```python
from build123d import *

# Parameters (mm, degrees)
SKETCH1_W           = 40
SKETCH1_H           = 25
BOSS_EXTRUDE1_DEPTH = 2
SKETCH2_W           = 25
SKETCH2_H           = 2
BOSS_EXTRUDE2_DEPTH = 2
SKETCH3_W           = 13
SKETCH3_H           = 17
CUT_EXTRUDE1_DEPTH  = 3
SKETCH4_R           = 0.6
BOSS_EXTRUDE3_DEPTH = 5
SKETCH5_W           = 16
SKETCH5_H           = 2
BOSS_EXTRUDE4_DEPTH = 4
SKETCH6_W           = 12
SKETCH6_H           = 2
CUT_EXTRUDE2_DEPTH  = 4
FILLET1_START       = -1
FILLET1_DEPTH       = 4
FILLET1_2_DEPTH     = 2
MIRROR4_DEPTH       = 2
FILLET2_R           = 2
FILLET3_R           = 2


with BuildPart() as part:
    # Sketch1 → Boss-Extrude1 (new body)
    with BuildSketch(Plane(origin=(0, 0, 0), x_dir=(1, 0, 0), z_dir=(0, 1, 0))):
        Rectangle(SKETCH1_W, SKETCH1_H)
    extrude(amount=BOSS_EXTRUDE1_DEPTH)

    # Sketch2 → Boss-Extrude2 (add)
    with BuildSketch(Plane(origin=(0, 2, 0), x_dir=(1, 0, 0), z_dir=(0, 1, 0))):
        with Locations((-7.5, 11.5)):
            Rectangle(SKETCH2_W, SKETCH2_H)
    boss_extrude2 = extrude(amount=BOSS_EXTRUDE2_DEPTH)

    # Mirror1: Boss-Extrude2 across plane
    add(boss_extrude2.mirror(Plane.XY))

    # Sketch3 → Cut-Extrude1 (cut)
    with BuildSketch(Plane(origin=(0, 2, 0), x_dir=(1, 0, 0), z_dir=(0, 1, 0))):
        with Locations((13.5, 0)):
            Rectangle(SKETCH3_W, SKETCH3_H)
    extrude(amount=-CUT_EXTRUDE1_DEPTH, mode=Mode.SUBTRACT)

    # Sketch4 → Boss-Extrude3 (add)
    with BuildSketch(Plane(origin=(0, 2, 0), x_dir=(1, 0, 0), z_dir=(0, 1, 0))):
        with Locations(Location((18.188184095, -10.67, 0), (0, 0, 270))):
            Circle(SKETCH4_R)
    boss_extrude3 = extrude(amount=BOSS_EXTRUDE3_DEPTH)

    # Mirror2: Boss-Extrude3 across plane
    add(boss_extrude3.mirror(Plane.XY))

    # Sketch5 → Boss-Extrude4 (add)
    with BuildSketch(Plane.XY.offset(12.5)):
        with Locations((0, 1)):
            Rectangle(SKETCH5_W, SKETCH5_H)
    extrude(amount=BOSS_EXTRUDE4_DEPTH)

    # Sketch6 → Cut-Extrude2 (cut)
    with BuildSketch(Plane(origin=(0, 2, 0), x_dir=(1, 0, 0), z_dir=(0, 1, 0))):
        with Locations((0, -13.5)):
            Rectangle(SKETCH6_W, SKETCH6_H)
    extrude(amount=-CUT_EXTRUDE2_DEPTH, mode=Mode.SUBTRACT)

    # Fillet1: read off the stored shape, not the designer's step
    # Fillet1 outline → Fillet1 (cut)
    with BuildSketch(Plane(origin=(0, 0, 0), x_dir=(1, 0, 0), z_dir=(0, 1, 0)).offset(FILLET1_START)):
        with BuildLine():
            ThreePointArc((8, -14.5), (7.414213562, -15.914213562), (6, -16.5))
            Line((6, -16.5), (8, -16.5))
            Line((8, -16.5), (8, -14.5))
        make_face()
        with BuildLine():
            Line((-8, -16.5), (-6, -16.5))
            ThreePointArc((-6, -16.5), (-7.414213562, -15.914213562), (-8, -14.5))
            Line((-8, -14.5), (-8, -16.5))
        make_face()
    extrude(amount=FILLET1_DEPTH, mode=Mode.SUBTRACT)

    # Fillet1 2 outline → Fillet1 2 (add)
    with BuildSketch(Plane(origin=(0, 0, 0), x_dir=(1, 0, 0), z_dir=(0, 1, 0))):
        with BuildLine():
            Line((8, -12.5), (8, -14.5))
            ThreePointArc((8, -14.5), (8.585786438, -13.085786438), (10, -12.5))
            Line((10, -12.5), (8, -12.5))
        make_face()
        with BuildLine():
            ThreePointArc((-10, -12.5), (-8.585786438, -13.085786438), (-8, -14.5))
            Line((-8, -14.5), (-8, -12.5))
            Line((-8, -12.5), (-10, -12.5))
        make_face()
    extrude(amount=FILLET1_2_DEPTH)

    # Mirror4: read off the stored shape, not the designer's step
    # Mirror4 outline → Mirror4 (add)
    with BuildSketch(Plane(origin=(0, 0, 0), x_dir=(1, 0, 0), z_dir=(0, 1, 0))):
        with BuildLine():
            Line((-8, 12.5), (-6, 12.5))
            Line((-6, 12.5), (-6, 14.5))
            Line((-6, 14.5), (6, 14.5))
            Line((6, 14.5), (6, 12.5))
            Line((6, 12.5), (8, 12.5))
            Line((8, 12.5), (8, 14.5))
            ThreePointArc((8, 14.5), (7.414213562, 15.914213562), (6, 16.5))
            Line((6, 16.5), (-6, 16.5))
            ThreePointArc((-6, 16.5), (-7.414213562, 15.914213562), (-8, 14.5))
            Line((-8, 14.5), (-8, 12.5))
        make_face()
    extrude(amount=MIRROR4_DEPTH)

    # Fillet2
    # the kernel refuses this fillet: 2 mm, written as the material it adds along each edge
    with BuildSketch(Plane(origin=(-8, 0, -12.5), x_dir=(-1, 0, 0), z_dir=(0, 1, 0))) as fillet2_piece_1:
        with BuildLine():
            CenterArc((FILLET2_R, -FILLET2_R), FILLET2_R, 90, 90)
            Line((0, -FILLET2_R), (0, 0))
            Line((0, 0), (FILLET2_R, 0))
        make_face()
    extrude(amount=2)
    with BuildSketch(Plane(origin=(8, 0, -12.5), x_dir=(1, 0, 0), z_dir=(0, 1, 0))) as fillet2_piece_2:
        with BuildLine():
            CenterArc((FILLET2_R, FILLET2_R), FILLET2_R, 180, 90)
            Line((0, FILLET2_R), (0, 0))
            Line((0, 0), (FILLET2_R, 0))
        make_face()
    extrude(amount=2)

    # Fillet3
    fillet3_edges = [part.edges().sort_by_distance(p)[0] for p in [
        (7, 1, 8.5),
        (7, 1, -8.5),
    ]]
    fillet(fillet3_edges, radius=FILLET3_R)


solid = part.part
```
Design review of the part built by this model. Coordinates are the model's own, in mm. A direction names the side the tool comes from. Round coordinates to 2 decimals unless told otherwise and drop trailing zeros. Write each loop counter-clockwise with the first axis right and the second up, starting at its lowest first coordinate (ties: lowest second). Pieces come first, ordered by that corner, then holes.
Item 1: Clearance check with flat-ended pins moving along their axes: pin 1 Ø1.6 at (y, z) = (3.5, -11.5) entering from +X; pin 2 Ø1 at (x, y) = (15.5, 1.5) entering from -Z; pin 3 Ø1 at (x, z) = (-5.5, 9.5) entering from +Y; pin 4 Ø4 at (y, z) = (3, 3.5) entering from -X. State where each tip first meets the part, or that it passes through.
Item 2: We need section B-B on y = 1.5. State how many separate pieces and enclosed holes the cut face has, and give its area (3 significant figures).
Item 3: For faces 4 (the flat face through (-6, 1, -13)), 5 (the flat face through (-8, 4, -12)), 6 (the flat face through (-8, 3, 10.5)), 7 (the cylindrical face through (18.783, 4.465, -10.592)), 8 (the flat face through (7, 1, 0)), list the 3-axis set-ups (+Z, -Z, +X, -X, +Y, -Y) from which the entire face can be reached by the end or side of a thin tool; tool diameter is ignored.
Item 4: The part is to be moulded in two halves that separate along Z. For faces 1 (the flat face through (15, 1, -12.5)), 2 (the flat face through (-4, 2, 0)), 3 (the flat face through (20, 1, 11)), say which applies: +Z half, -Z half, draft (parallel to the pull), parting line (faces both ways), or undercut.
Item 5: We need section A-A on x = -5. Write out the cut boundary in (y, z), and give its area (3 significant figures).
Item 6: For probe 1 along Z at (x, y) = (2.5, 0.75); probe 2 along Z at (x, y) = (-11, 3.75); probe 3 along Y at (x, z) = (0, 12), list the stretches that pass through material, from the lowest coordinate up.
Item 7: We need section D-D on x = 8.5. Write out the cut boundary in (y, z), and give its area (3 significant figures).
Item 8: We need section C-C on z = 14. Write out the cut boundary in (x, y), and give its area (3 significant figures).
Returned:
1. pin 1: stops at x = 18.79
1. pin 2: stops at z = -12.5
1. pin 3: stops at y = 2
1. pin 4: stops at x = -20
2. separate pieces: 1
2. enclosed holes: 2
2. area: 861 mm2
3. face 4: +Y, -Y
3. face 5: +Z, -Z, -X, +Y
3. face 6: -X, +Y
3. face 7: +Y
3. face 8: +X, +Y, -Y
4. face 1: -Z half
4. face 2: undercut
4. face 3: draft
5. outline: (0, -16.5) - (2, -16.5) - (2, -14.5) - (0, -14.5) - close; (0, -12.5) - (4, -12.5) - (4, -10.5) - (2, -10.5) - (2, 10.5) - (4, 10.5) - (4, 12.5) - (0, 12.5) - close; (0, 14.5) - (2, 14.5) - (2, 16.5) - (0, 16.5) - close
5. area: 66.0 mm2
6. probe 1: z = -16.5 to -14.5, -12.5 to 12.5, 14.5 to 16.5
6. probe 2: z = -12.5 to -10.5, 10.5 to 12.5
6. probe 3: y = 0 to 4
7. outline: (0, -13.18) - (2, -13.18) - (2, -8.44) - (0, -8.44) - close; (0, 8.44) - (2, 8.44) - (2, 13.18) - (0, 13.18) - close
7. area: 19.0 mm2
8. outline: (-8.06, 0) - (-6, 0) - (-6, 2) - (-8.06, 2) - close; (6, 0) - (8.06, 0) - (8.06, 2) - (6, 2) - close
8. area: 8.25 mm2
